```python
from build123d import *

# Parameters (mm, degrees)
F1_DEPTH  = 20
F2_DEPTH  = 12
F3_DEPTH  = 10
F4_DEPTH  = 10
F5_W      = 25
F5_H      = 20
F6_DEPTH  = 14
F7_SIZE   = 10
F8_SIZE   = 6.99999
F9_DEPTH  = 10
F10_W     = 17
F10_H     = 80
F11_DEPTH = 20.001
F13_DEPTH = 20


# Not quite as in the source:
# - a fillet or chamfer is up to 0.001 mm smaller than in the source, because OpenCascade refuses the exact size
# - a feature names something its author has since deleted; it is built from what else it names


with BuildPart() as f1:
    # F0 (on Top) → F1 (new body)
    with BuildSketch(Plane.XY):
        Polygon((78, -43.2), (75, -45), (78, -45), align=None)
        Polygon((33.3333333333, -20), (0, 0), (0, -90), (33.3333333333, -70), (25, -70), (25, -20), align=None)
        Polygon((150, -90), (150, 0), (116.6666666667, -20), (125, -20), (125, -70), (116.6666666667, -70), align=None)
        Polygon((75, 0), (0, 0), (33.3333333333, -20), (35, -20), (35, -14), (42, -14), (42, -6), (45, -6), (45, -14), (72, -14), (72, -43.2), (75, -45), align=None)
        Polygon((150, 0), (75, 0), (75, -45), (78, -43.2), (78, -14), (105, -14), (105, -6), (108, -6), (108, -14), (115, -14), (115, -20), (116.6666666667, -20), align=None)
        Polygon((78, -45), (75, -45), (78, -46.8), align=None)
        Polygon((72, -45), (75, -45), (72, -43.2), align=None)
        Polygon((72, -46.8), (75, -45), (72, -45), align=None)
        Polygon((78, -46.8), (75, -45), (75, -90), (150, -90), (116.6666666667, -70), (115, -70), (115, -69), (105, -63), (91.6666666667, -55), (85, -55), (85, -62), (78, -62), (78, -55), (78, -48), align=None)
        Polygon((33.3333333333, -70), (0, -90), (75, -90), (75, -45), (72, -46.8), (72, -48), (72, -55), (72, -62), (65, -62), (65, -55), (58.3333333333, -55), (45, -63), (35, -69), (35, -70), align=None)
        Polygon((35, -55), (35, -69), (45, -63), (42, -63), (42, -55), align=None)
        Polygon((45, -63), (58.3333333333, -55), (45, -55), align=None)
        Polygon((105, -55), (91.6666666667, -55), (105, -63), align=None)
        Polygon((105, -63), (115, -69), (115, -55), (108, -55), (108, -63), align=None)
    extrude(amount=F1_DEPTH)

    # F2 (cut): a face of the model
    f2_faces = [f1.faces().sort_by_distance(p)[0] for p in [
        (75, -90, 10),
    ]]
    extrude(f2_faces, amount=-F2_DEPTH, mode=Mode.SUBTRACT)

    # F3 (cut): a face of the model
    f3_faces = [f1.faces().sort_by_distance(p)[0] for p in [
        (150, -39, 10),
    ]]
    extrude(f3_faces, amount=-F3_DEPTH, mode=Mode.SUBTRACT)

    # F4 (cut): a face of the model
    f4_faces = [f1.faces().sort_by_distance(p)[0] for p in [
        (0, -39, 10),
    ]]
    extrude(f4_faces, amount=-F4_DEPTH, mode=Mode.SUBTRACT)

    # F5 (on face) → F6 (cut)
    with BuildSketch(Plane.XZ.offset(78)):
        with Locations((87.5, 10)):
            Rectangle(F5_W, F5_H)
        with Locations((62.5, 10)):
            Rectangle(F5_W, F5_H)
    extrude(amount=-F6_DEPTH, mode=Mode.SUBTRACT)

    # F7
    f7_edges = [f1.edges().sort_by_distance(p)[0] for p in [
        (100, -78, 10),
        (50, -78, 10),
    ]]
    chamfer(f7_edges, length=F7_SIZE)

    # F8 (size 7 in the source; OpenCascade refuses exactly that, so slightly less here)
    f8_edges = [f1.edges().sort_by_distance(p)[0] for p in [
        (85, -55, 10),
        (65, -55, 10),
    ]]
    chamfer(f8_edges, length=F8_SIZE)

    # F9 (add): a face of the model
    f9_faces = [f1.faces().sort_by_distance(p)[0] for p in [
        (75, 0, 10),
    ]]
    extrude(f9_faces, amount=F9_DEPTH)

    # F10 (on face) → F11 (cut, through all)
    with BuildSketch(Plane.XY.offset(20)):
        with Locations((26.5, -38)):
            Rectangle(F10_W, F10_H)
        with Locations((123.5, -38)):
            Rectangle(F10_W, F10_H)
    extrude(amount=-F11_DEPTH, mode=Mode.SUBTRACT)

    # F12 (on face) → F13 (join)
    with BuildSketch(Plane.XY.offset(20)):
        Polygon((18, -88), (18, -78), (10, -78), (10, -94), (40, -94), (40, -78), (35, -78), (35, -88), align=None)
        Polygon((140, -94), (140, -78), (132, -78), (132, -88), (115, -88), (115, -78), (110, -78), (110, -94), align=None)
    extrude(amount=-F13_DEPTH)


solid = f1.part
```
Geometry check sheet. Reference: the model listing, model coordinates, mm. Give positions to 0.01 mm unless a question says otherwise; leave off trailing zeros. Loops run counter-clockwise (first coordinate to the right, second up) from the corner with the lowest first, then second, coordinate; pieces in that order, holes last. Notation, with made-up numbers: (76.5, 25.5) - (121.5, 25.5) arc R20 ccw to (121.5, 48.5) - close; hole circle Ø5 at (1, 84.25). An arc over 180 degrees is marked (long way). Use CSV: the item, a comma, the result in double quotes. Start each with the question number.
Q1. Section check C-C, the plane x = 61. Record the cut outline in (y, z), and give its area (3 significant figures).
Q2. Scan lines: probe 1 along X at (y, z) = (-66, 18.5); probe 2 along X at (y, z) = (-24.5, 17); probe 3 along Y at (x, z) = (70, 11.75). Record each from-to range of solid material in increasing order. Write a range as from..to.
Q3. Go/stop test with a flat-tipped pin: pin 1 Ø5 at (x, z) = (59, 11.5) entering from -Y. Record where the tip stops, or that it passes through.
Q4. Section check D-D, the plane z = 10.5. Count the separate pieces of the cut face and the enclosed holes in it, and give its area (3 significant figures).
Q5. Release check for a two-part mould opening along Y. For faces 1 (the face through (42, -59, 10)), 2 (the face through (76, 10, 10)) record: +Y half, -Y half, draft (parallel to the pull), parting line (faces both ways), or undercut.
Q6. Section check B-B, the plane y = -43. Record the cut outline in (x, z).
Findings below:
1,outline,"(-64, 0) - (-58, 0) - (-58, 20) - (-64, 20) - close; (-14, 0) - (10, 0) - (10, 20) - (-14, 20) - close"
1,area,"600 mm^2"
2,probe 1,"x = 10..18, 35..50, 100..115, 132..140"
2,probe 2,"x = 10..18, 72..78, 132..140"
2,probe 3,"y = -64..-62, -14..10"
3,pin 1,"stops at y = -64"
4,separate pieces,"1"
4,enclosed holes,"2"
4,area,"5,260 mm^2"
5,face 1,"undercut"
5,face 2,"+Y half"
6,outline,"(10, 0) - (18, 0) - (18, 20) - (10, 20) - close; (72, 0) - (78, 0) - (78, 20) - (72, 20) - close; (132, 0) - (140, 0) - (140, 20) - (132, 20) - close"
